Here's the drawing with two shaded views (mm, measured from the low corner). I have some questions. Round coordinates to 2 decimals unless told otherwise and drop trailing zeros. Write each loop counter-clockwise with the first axis right and the second up, starting at its lowest first coordinate (ties: lowest second). Pieces come first, ordered by that corner, then holes. Notation, with made-up numbers: (54.5, 55.5) -> (109.5, 55.5) arc R20 ccw to (109.5, 89.5) -> close; hole circle Ø3 at (-25, -5.75). An arc over 180 degrees is marked (long way). Use CSV: the item, a comma, the result in double quotes.
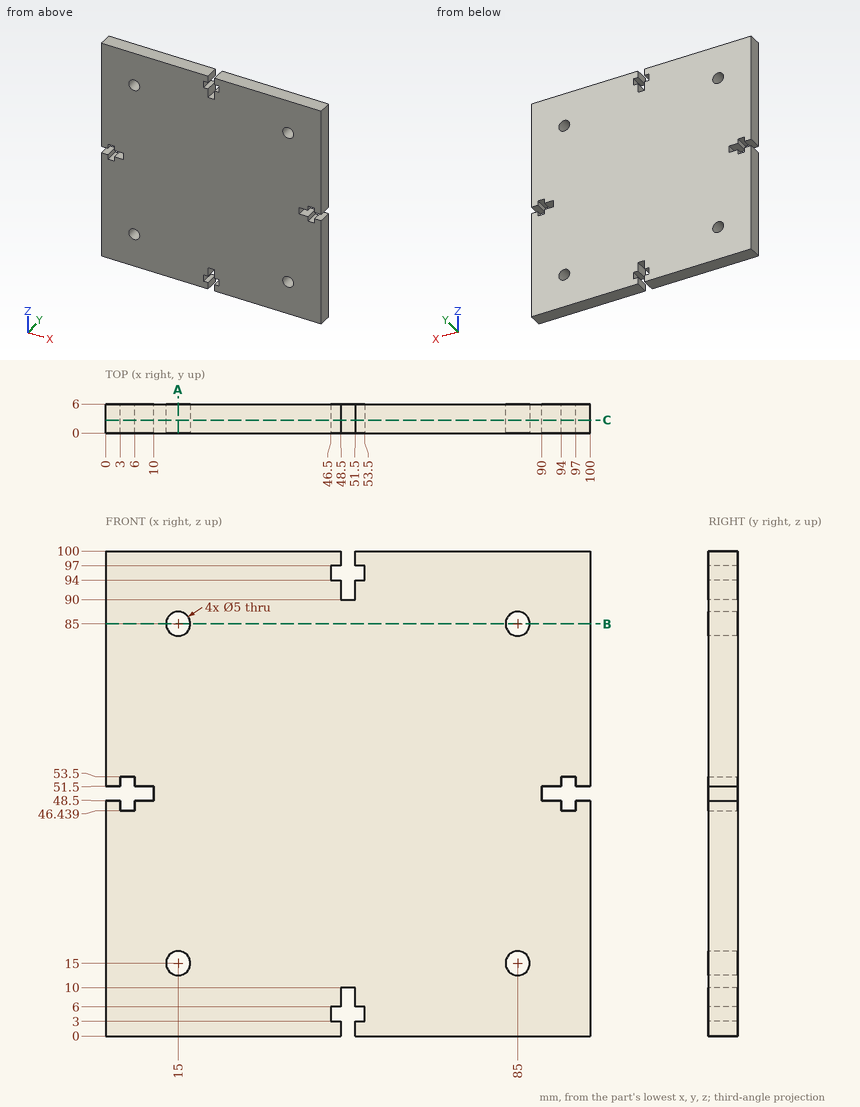
Q1. Suppose I cut it at A-A (x = 15). Write out the boundary of the cut face in (y, z), and give its area (3 significant figures).
Resolved:
outline,"(0, 0) -> (6, 0) -> (6, 12.5) -> (0, 12.5) -> close; (0, 17.5) -> (6, 17.5) -> (6, 82.5) -> (0, 82.5) -> close; (0, 87.5) -> (6, 87.5) -> (6, 100) -> (0, 100) -> close"
area,"540 mm^2"
Q2. Suppose I cut it at C-C (y = 2.7). Count the separate pieces of the cut face and the enclosed holes in it, and give its area (3 significant figures).
Resolved:
separate pieces,"1"
enclosed holes,"4"
area,"9,750 mm^2"
Q3. Suppose I cut it at B-B (z = 85). Write out the boundary of the cut face in (x, y), and give its area (3 significant figures).
Resolved:
outline,"(0, 0) -> (12.5, 0) -> (12.5, 6) -> (0, 6) -> close; (17.5, 0) -> (82.5, 0) -> (82.5, 6) -> (17.5, 6) -> close; (87.5, 0) -> (100, 0) -> (100, 6) -> (87.5, 6) -> close"
area,"540 mm^2"
Q4. Please list where these lines run through material, in increasing order: probe 1 along X at (y, z) = (1.4, 85); probe 2 along Z at (x, y) = (52, 5.45).
Resolved:
probe 1,"x = 0 to 12.5, 17.5 to 82.5, 87.5 to 100"
probe 2,"z = 0 to 3, 6 to 94, 97 to 100"
Q5. Will this pin go through, and if not, where does the flat tip stop? P1, Ø4, axis at x = 15, z = 15, coming from the +Y side.
Resolved:
P1,"passes through"
